from build123d import *

# Parameters (mm, degrees)
SKETCH_1_W             = 23.5
SKETCH_1_H             = 12
EXTRUDE_1_DEPTH        = 76
HOLE_WIZARD_M6_1_D     = 5
HOLE_WIZARD_M6_1_DEPTH = 15
HOLE_WIZARD_M6_1_TIP   = 1.502151548
HOLE_WIZARD_M6_2_D     = 5
HOLE_WIZARD_M6_2_DEPTH = 15
HOLE_WIZARD_M6_2_TIP   = 1.502151548


with BuildPart() as part:
    # 草图1 → 凸台-拉伸1 (new, symmetric)
    with BuildSketch(Plane(origin=(0, 0, 0), x_dir=(0, 0, -1), z_dir=(1, 0, 0))):
        with BuildLine():
            Line((-14, 15), (-11.5, 15))
            Line((-11.5, 15), (-11.5, 13.5))
            Line((-11.5, 13.5), (-11.4, 13.5))
            ThreePointArc((-11.4, 13.5), (-11.117157288, 13.382842712), (-11, 13.1))
            Line((-11, 13.1), (-11, 12))
            Line((-11, 12), (-9.5, 12))
            Line((-9.5, 12), (-9.5, 15))
            Line((-9.5, 15), (-8, 15))
            Line((-8, 15), (-8, 12.5))
            Line((-8, 12.5), (-5, 12.5))
            Line((-5, 12.5), (-5, 15))
            Line((-5, 15), (5, 15))
            Line((5, 15), (5, 12.5))
            Line((5, 12.5), (8, 12.5))
            Line((8, 12.5), (8, 15))
            Line((8, 15), (9.5, 15))
            Line((9.5, 15), (9.5, 12))
            Line((9.5, 12), (11, 12))
            Line((11, 12), (11, 13.1))
            ThreePointArc((11, 13.1), (11.117157288, 13.382842712), (11.4, 13.5))
            Line((11.4, 13.5), (11.5, 13.5))
            Line((11.5, 13.5), (11.5, 15))
            Line((11.5, 15), (14, 15))
            ThreePointArc((14, 15), (14.707106781, 14.707106781), (15, 14))
            Line((15, 14), (15, 8))
            Line((15, 8), (12.5, 8))
            Line((12.5, 8), (12.5, 5))
            Line((12.5, 5), (15, 5))
            Line((15, 5), (15, -5))
            Line((15, -5), (12.5, -5))
            Line((12.5, -5), (12.5, -8))
            Line((12.5, -8), (15, -8))
            Line((15, -8), (15, -14))
            ThreePointArc((15, -14), (14.707106781, -14.707106781), (14, -15))
            Line((14, -15), (11.5, -15))
            Line((11.5, -15), (11.5, -13.5))
            Line((11.5, -13.5), (11.4, -13.5))
            ThreePointArc((11.4, -13.5), (11.117157288, -13.382842712), (11, -13.1))
            Line((11, -13.1), (11, -12))
            Line((11, -12), (9.5, -12))
            Line((9.5, -12), (9.5, -15))
            Line((9.5, -15), (8, -15))
            Line((8, -15), (8, -12.5))
            Line((8, -12.5), (5, -12.5))
            Line((5, -12.5), (5, -15))
            Line((5, -15), (-5, -15))
            Line((-5, -15), (-5, -12.5))
            Line((-5, -12.5), (-8, -12.5))
            Line((-8, -12.5), (-8, -15))
            Line((-8, -15), (-9.5, -15))
            Line((-9.5, -15), (-9.5, -12))
            Line((-9.5, -12), (-11, -12))
            Line((-11, -12), (-11, -13.1))
            ThreePointArc((-11, -13.1), (-11.117157288, -13.382842712), (-11.4, -13.5))
            Line((-11.4, -13.5), (-11.5, -13.5))
            Line((-11.5, -13.5), (-11.5, -15))
            Line((-11.5, -15), (-14, -15))
            ThreePointArc((-14, -15), (-14.707106781, -14.707106781), (-15, -14))
            Line((-15, -14), (-15, 14))
            ThreePointArc((-15, 14), (-14.707106781, 14.707106781), (-14, 15))
        make_face()
        with BuildLine():
            Line((12, -10.5), (12, -8.5))
            ThreePointArc((12, -8.5), (11.853553391, -8.146446609), (11.5, -8))
            Line((11.5, -8), (-11.5, -8))
            ThreePointArc((-11.5, -8), (-11.853553391, -8.146446609), (-12, -8.5))
            Line((-12, -8.5), (-12, -10.5))
            ThreePointArc((-12, -10.5), (-11.853553391, -10.853553391), (-11.5, -11))
            Line((-11.5, -11), (11.5, -11))
            ThreePointArc((11.5, -11), (11.853553391, -10.853553391), (12, -10.5))
        make_face(mode=Mode.SUBTRACT)
        with BuildLine():
            Line((-11.5, 11), (11.5, 11))
            ThreePointArc((11.5, 11), (11.853553391, 10.853553391), (12, 10.5))
            Line((12, 10.5), (12, 8.5))
            ThreePointArc((12, 8.5), (11.853553391, 8.146446609), (11.5, 8))
            Line((11.5, 8), (-11.5, 8))
            ThreePointArc((-11.5, 8), (-11.853553391, 8.146446609), (-12, 8.5))
            Line((-12, 8.5), (-12, 10.5))
            ThreePointArc((-12, 10.5), (-11.853553391, 10.853553391), (-11.5, 11))
        make_face(mode=Mode.SUBTRACT)
        Rectangle(SKETCH_1_W, SKETCH_1_H, mode=Mode.SUBTRACT)
    extrude(amount=EXTRUDE_1_DEPTH, both=True)

    # M6 螺纹孔1
    with Locations(Plane(origin=(0, 0, -15), x_dir=(-1, 0, 0), z_dir=(0, 0, -1))):
        with Locations((-56, 0), (-41, 0), (41, 0), (56, 0)):
            Hole(HOLE_WIZARD_M6_1_D / 2, depth=HOLE_WIZARD_M6_1_DEPTH)
            with Locations((0, 0, -(HOLE_WIZARD_M6_1_DEPTH + HOLE_WIZARD_M6_1_TIP / 2))):  # 118° drill point
                Cone(0, HOLE_WIZARD_M6_1_D / 2, HOLE_WIZARD_M6_1_TIP, mode=Mode.SUBTRACT)

    # M6 螺纹孔2
    with Locations(Plane.XZ.offset(15)):
        with Locations((56, 0), (41, 0), (-41, 0), (-56, 0)):
            Hole(HOLE_WIZARD_M6_2_D / 2, depth=HOLE_WIZARD_M6_2_DEPTH)
            with Locations((0, 0, -(HOLE_WIZARD_M6_2_DEPTH + HOLE_WIZARD_M6_2_TIP / 2))):  # 118° drill point
                Cone(0, HOLE_WIZARD_M6_2_D / 2, HOLE_WIZARD_M6_2_TIP, mode=Mode.SUBTRACT)


solid = part.part
Can you work these out from the model? Positions are in its coordinate system, mm. A direction names the side the tool comes from. Round coordinates to 2 decimals unless told otherwise and drop trailing zeros. Write each loop counter-clockwise with the first axis right and the second up, starting at its lowest first coordinate (ties: lowest second). Pieces come first, ordered by that corner, then holes. Notation, with made-up numbers: M 60,46.25 L 75,46.25 A11 cw 75,63.25 Z; hole C -22.75,76.5 d11. An arc over 180 degrees is marked long. Use CSV: the item, a comma, the result in double quotes.
(1) On a 3-axis mill with a long thin cutter (end or side, diameter ignored), from which of +Z, -Z, +X, -X, +Y, -Y can I reach the whole of each face in a straight line? I mean faces 5 (the flat face through (1, -8, 0)), 6 (the flat face through (1, 8, -14)), 7 (the flat face through (1, 14, -5)). Say none if no direction works.
Check values:
face 5,"+X, -X"
face 6,"-Z, +X, -X"
face 7,"+X, -X, +Y"
(2) I need wall thicknesses on line 1 along Z through (x, y) = (56, -13.05); line 2 along Y through (x, z) = (22.5, 5.25); line 3 along Y through (x, z) = (-56, -14). Which ranges of each line are inside material? Lowest first, please.
Check values:
line 1,"-15 to -11, -9.5 to -8, -5 to -2.5, 2.5 to 5, 8 to 9.5, 11 to 15"
line 2,"-12.5 to -11, -8 to -6, 6 to 8, 11 to 12.5"
line 3,"-15 to -8, -5 to -2.5, 2.5 to 5, 8 to 15"
(3) We'd pull the mould along Y, two halves only. Please class faces 1 (the flat face through (1, 11, 0)), 2 (the cylindrical face through (-58.31, -6.99, -0.96)), 3 (the flat face through (1, 15, 13)), 4 (the flat face through (1, 0, 11.75)): +Y half, -Y half, draft (parallel to the pull), parting line (faces both ways), or undercut.
Check values:
face 1,"undercut"
face 2,"draft"
face 3,"+Y half"
face 4,"undercut"
(4) I'm going to push flat-ended pins straight in: pin 1 (3 mm diameter, centred on x = -56, z = 0, fed in from -Y); pin 2 (3 mm diameter, centred on x = 56, y = 0, fed in from -Z). Where does each tip first touch, or does it pass through?
Check values:
pin 1,"y = 6"
pin 2,"z = 11.75"
(5) Imagine slicing it at A-A (y = 0). Write out the boundary of the cut face in (x, z).
Check values:
outline,"M -76,-15 L -58.5,-15 L -58.5,-11.75 L -76,-11.75 Z; M -76,11.75 L 76,11.75 L 76,15 L -76,15 Z; M -53.5,-15 L -43.5,-15 L -43.5,-11.75 L -53.5,-11.75 Z; M -38.5,-15 L 38.5,-15 L 38.5,-11.75 L -38.5,-11.75 Z; M 43.5,-15 L 53.5,-15 L 53.5,-11.75 L 43.5,-11.75 Z; M 58.5,-15 L 76,-15 L 76,-11.75 L 58.5,-11.75 Z"
(6) Imagine slicing it at B-B (x = 41). Count the separate pieces of the cut face and the enclosed holes in it, plus the area to 3 significant figures.
Check values:
separate pieces,"2"
enclosed holes,"1"
area,"361 mm^2"
